Part model, mm, in its own coordinate system. Give positions to 0.01 mm unless a question says otherwise; leave off trailing zeros. Write each loop counter-clockwise with the first axis right and the second up, starting at its lowest first coordinate (ties: lowest second). Pieces come first, ordered by that corner, then holes. Notation, with made-up numbers: M -19,88.25 L 18,88.25 A12 cw 18,100.25 Z; hole C -40,11 d8. An arc over 180 degrees is marked long. Use CSV: the item, a comma, the result in double quotes. Start each with the question number.
1. Drill centre lines: line 1 along Y through (x, z) = (-80.5, -3.75); line 2 along X through (y, z) = (38, -4.25); line 3 along X through (y, z) = (0, -3.9). Where is each one in solid material? Low to high. Write a range as from..to.
2. Band-saw the part on A-A, the plane y = 25.4. List the corners of the cut face in (x, z), then the cut area to 3 significant figures.
3. Drop flat-ended pins along their axis: pin 1 Ø2 at (x, y) = (-89, -20) entering from +Z; pin 2 Ø3 at (x, y) = (-105.84, 25.4) entering from +Z. Give the stop position or say it passes through.
4. Band-saw the part on C-C, the plane z = -4.5. Count the separate pieces of the cut face and the enclosed holes in it, then the cut area to 3 significant figures.
5. Mould opens along X. For faces 1 (the face through (-32.815, -1, -3)), 2 (the face through (-92, 1, 0)), 3 (the face through (-107.03, 25.78, -4.26)) say: pulls with the +X half, pulls with the -X half, needs draft (parallel to the pull), parting line crosses it, or undercut.
6. Band-saw the part on B-B, the plane y = 38.1. List the corners of the cut face in (x, z), then the cut area to 3 significant figures.
from build123d import *

# Parameters (mm, degrees)
F1_DEPTH       = 6.35
F2_D           = 6.6
F2_DEPTH       = 12.7
F2_TIP         = 1.9828400428
F3_D           = 2.5
F3_DEPTH       = 12.7014
F3_CSINK_D     = 6.72
F3_CSINK_ANGLE = 90
F3_TIP         = 0.7510757738


with BuildPart() as f1:
    # F0 (on Top) → F1 (new body)
    with BuildSketch(Plane.XY):
        Polygon((-32.8152788184, 50.8), (-128.0652788184, 50.8), (-128.0652788184, -50.8), (-96.3170453906, -50.8), (-32.8152788184, -50.8), align=None)
    extrude(amount=-F1_DEPTH)

    # F2
    with Locations(Plane.XY):
        with Locations((-115.3652788184, 38.1), (-45.5152788184, 38.1), (-45.5152788184, -38.1), (-115.3652788184, -38.1)):
            Hole(F2_D / 2, depth=F2_DEPTH)
            with Locations((0, 0, -(F2_DEPTH + F2_TIP / 2))):  # 118° drill point
                Cone(0, F2_D / 2, F2_TIP, mode=Mode.SUBTRACT)

    # F3
    with Locations(Plane.XY):
        with Locations((-105.8402788184, 25.4), (-80.4402788184, 25.4), (-55.0402788184, 25.4), (-80.4402788184, 0), (-55.0402788184, 0), (-105.8402788184, 0), (-105.8402788184, -25.4), (-80.4402788184, -25.4), (-55.0402788184, -25.4)):
            CounterSinkHole(F3_D / 2, F3_CSINK_D / 2, depth=F3_DEPTH, counter_sink_angle=F3_CSINK_ANGLE)
            with Locations((0, 0, -(F3_DEPTH + F3_TIP / 2))):  # 118° drill point
                Cone(0, F3_D / 2, F3_TIP, mode=Mode.SUBTRACT)


solid = f1.part
Output:
1,line 1,"y = -50.8..-26.65, -24.15..-1.25, 1.25..24.15, 26.65..50.8"
1,line 2,"x = -128.07..-118.66, -112.07..-48.81, -42.22..-32.82"
1,line 3,"x = -128.07..-107.09, -104.59..-81.69, -79.19..-56.29, -53.79..-32.82"
2,outline,"M -128.07,-6.35 L -107.09,-6.35 L -107.09,-2.11 L -109.2,0 L -128.07,0 Z; M -104.59,-6.35 L -81.69,-6.35 L -81.69,-2.11 L -83.8,0 L -102.48,0 L -104.59,-2.11 Z; M -79.19,-6.35 L -56.29,-6.35 L -56.29,-2.11 L -58.4,0 L -77.08,0 L -79.19,-2.11 Z; M -53.79,-6.35 L -32.82,-6.35 L -32.82,0 L -51.68,0 L -53.79,-2.11 Z"
2,area,"544 mm²"
3,pin 1,"stops at z = 0"
3,pin 2,"stops at z = -1.86"
4,separate pieces,"1"
4,enclosed holes,"13"
4,area,"9,500 mm²"
5,face 1,"pulls with the +X half"
5,face 2,"needs draft"
5,face 3,"undercut"
6,outline,"M -128.07,-6.35 L -118.67,-6.35 L -118.67,0 L -128.07,0 Z; M -112.07,-6.35 L -48.82,-6.35 L -48.82,0 L -112.07,0 Z; M -42.22,-6.35 L -32.82,-6.35 L -32.82,0 L -42.22,0 Z"
6,area,"521 mm²"
